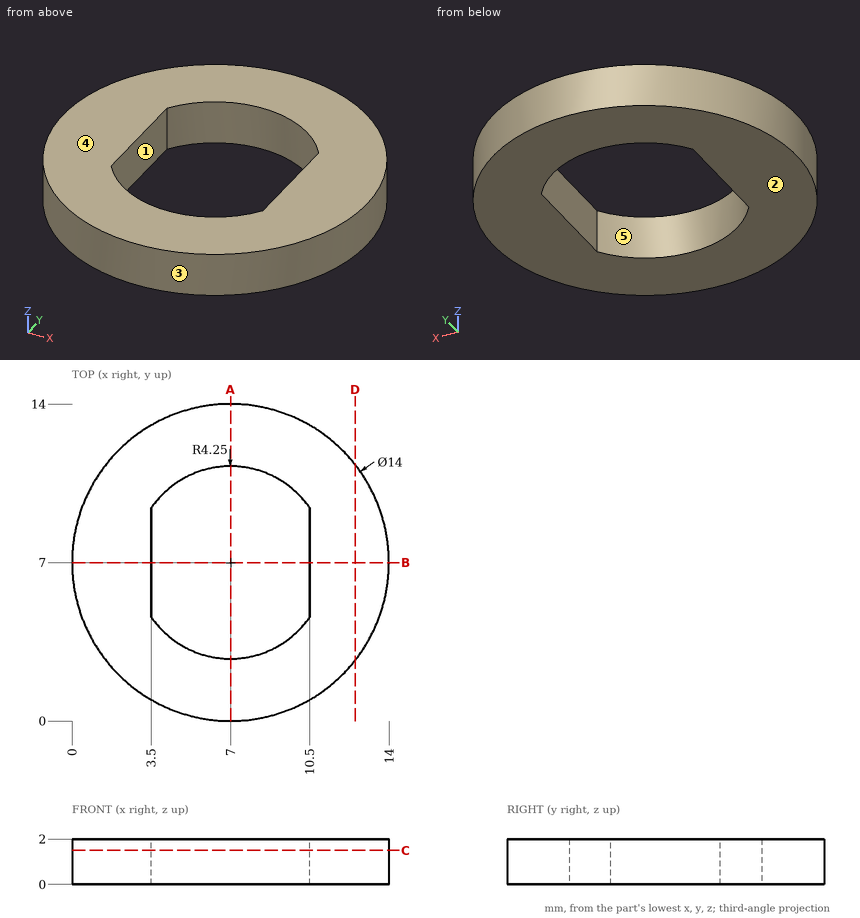
Verification items for this drawing (mm, ordinates from the low corner). A direction names the side the tool comes from. Coordinates: 2 decimals unless noted, no trailing zeros. Loops run counter-clockwise (first coordinate to the right, second up) from the corner with the lowest first, then second, coordinate; pieces in that order, holes last. Notation, with made-up numbers: (9.25, 59.5) - (60.25, 59.5) arc R21 cw to (60.25, 78.5) - close; hole circle Ø9 at (50.25, 62). An arc over 180 degrees is marked (long way). One line per item, written item: value. Start each with the question number.
(1) Cross-section at B-B on y = 7. Enter the section's corners in (x, z).
(2) Depth check by flat-ended pin: P1, Ø1, axis at y = 5.5, z = 1.5, coming from the +X side. Enter the tip coordinate at first touch or a pass-through.
(3) Cross-section at A-A on x = 7. Enter the section's corners in (y, z).
(4) Cross-section at D-D on x = 12.5. Enter the section's corners in (y, z).
(5) Material ranges on line 1 (Y direction, x = 5, z = 1.85); line 2 (Y direction, x = 7.75, z = 0.15); line 3 (X direction, y = 5.5, z = 0.6), recorded low to high. Write a range as [from, to].
(6) Tool access check on the marked faces 1 and 2. Record the directions out of +Z, -Z, +X, -X, +Y, -Y that give a thin tool (end or side, any length) a straight path to the whole face; none if there is none.
(7) Mould release check, pull along X, two halves, no side actions. Record for the marked faces 3, 4 and 5: released by +X, released by -X, zero draft, split by the parting line, or undercut.
(8) Cross-section at C-C on z = 1.5. Enter the section's corners in (x, y), plus the area to 3 significant figures.
Results below:
1. outline: (0, 0) - (3.5, 0) - (3.5, 2) - (0, 2) - close; (10.5, 0) - (14, 0) - (14, 2) - (10.5, 2) - close
2. P1: stops at x = 13.93
3. outline: (0, 0) - (2.75, 0) - (2.75, 2) - (0, 2) - close; (11.25, 0) - (14, 0) - (14, 2) - (11.25, 2) - close
4. outline: (2.67, 0) - (11.33, 0) - (11.33, 2) - (2.67, 2) - close
5. line 1: y = [0.29, 3.25], [10.75, 13.71]
5. line 2: y = [0.04, 2.82], [11.18, 13.96]
5. line 3: x = [0.16, 3.5], [10.5, 13.84]
6. face 1: +Z, -Z
6. face 2: -Z, +X, -X, +Y, -Y
7. face 3: split by the parting line
7. face 4: zero draft
7. face 5: undercut
8. outline: circle Ø14 at (7, 7); hole (3.5, 4.59) arc R4.25 ccw to (10.5, 4.59) - (10.5, 9.41) arc R4.25 ccw to (3.5, 9.41) - close
8. area: 102 mm2
